Geometry: final body of the model. Coordinates: model frame, mm. Face numbers are marked on the shaded views. Give positions to 0.01 mm unless a question says otherwise; leave off trailing zeros. Loops run counter-clockwise (first coordinate to the right, second up) from the corner with the lowest first, then second, coordinate; pieces in that order, holes last.
from build123d import *

# Parameters (mm, degrees)
SKETCH1_R          = 88.5571
SKETCH1_R_2        = 72.5043
SKETCH3_R          = 84.1375
CUT_EXTRUDE1_DEPTH = 44.45
SKETCH4_R          = 84.1375
CUT_EXTRUDE2_DEPTH = 44.45


with BuildPart() as part:
    # Sweep1: sweep along a path in Sketch2
    with BuildLine(Plane.XY) as sweep1_path:
        Line((0, 0), (50.8, 0))
        ThreePointArc((50.8, 0), (142.847625241, -38.127374759), (180.975, -130.175))
        Line((180.975, -130.175), (180.975, -180.975))
    # Sketch1 → Sweep1 (sweep)
    with BuildSketch(Plane(origin=(0, 0, 0), x_dir=(0, 0, -1), z_dir=(1, 0, 0))):
        Circle(SKETCH1_R)
        Circle(SKETCH1_R_2, mode=Mode.SUBTRACT)
    sweep(path=sweep1_path.line)

    # Sketch3 → Cut-Extrude1 (cut)
    with BuildSketch(Plane(origin=(0, -180.975, 0), x_dir=(-1, 0, 0), z_dir=(0, -1, 0))):
        with Locations((-180.975, 0)):
            Circle(SKETCH3_R)
    extrude(amount=-CUT_EXTRUDE1_DEPTH, mode=Mode.SUBTRACT)

    # Sketch4 → Cut-Extrude2 (cut)
    with BuildSketch(Plane.ZY):
        Circle(SKETCH4_R)
    extrude(amount=-CUT_EXTRUDE2_DEPTH, mode=Mode.SUBTRACT)


solid = part.part
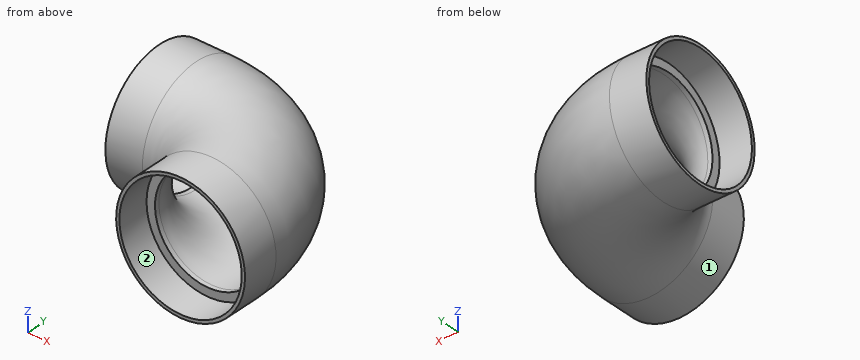
Item 1: Pin query (flat end, axial travel): pin 1 (2 mm diameter, centred on x = 38.5, y = -32.5, fed in from -Z); pin 2 (1.5 mm diameter, centred on x = 199, z = 55, fed in from +Y); pin 3 (4 mm diameter, centred on x = 162, z = 22, fed in from +Y). Return the tip coordinate at first contact, or that it passes through.
Values follow:
pin 1: stops at z = -82.77
pin 2: stops at y = 4.71
pin 3: stops at y = 56.27
Item 2: Draft query along Z for the marked faces 1 and 2. Return one class per face: +Z half, -Z half, draft (parallel to the pull), parting line (faces both ways), or undercut.
Values follow:
face 1: parting line
face 2: undercut
Item 3: Section query B-B on z = -5.5. Return loops of the section in (x, y) (3 decimals), plus the area to 3 significant figures.
Values follow:
outline: (0, -88.386) - (50.8, -88.386) arc R41.789 cw to (92.589, -130.175) - (92.589, -180.975) - (97.017, -180.975) - (97.017, -136.525) - (108.68, -136.525) - (108.68, -130.175) arc R57.88 ccw to (50.8, -72.295) - (44.45, -72.295) - (44.45, -83.958) - (0, -83.958) - close; (0, 83.958) - (44.45, 83.958) - (44.45, 72.295) - (50.8, 72.295) arc R202.47 cw to (253.27, -130.175) - (253.27, -136.525) - (264.933, -136.525) - (264.933, -180.975) - (269.361, -180.975) - (269.361, -130.175) arc R218.561 ccw to (50.8, 88.386) - (0, 88.386) - close
area: 7,780 mm2
Item 4: Ray query, probe 1 along Y at (x, z) = (46.25, 0); probe 2 along Y at (x, z) = (34, 0); probe 3 along X at (y, z) = (-131.75, 0). Return the intervals inside material, ascending.
Values follow:
probe 1: y = -88.56 to -72.5, 72.5 to 88.56
probe 2: y = -88.56 to -84.14, 84.14 to 88.56
probe 3: x = 92.42 to 108.47, 253.48 to 269.53
Item 5: Section query A-A on z = -52.5. Return loops of the section in (x, y) (3 decimals).
Values follow:
outline: (0, -71.317) - (50.8, -71.317) arc R58.858 cw to (109.658, -130.175) - (109.658, -180.975) - (115.226, -180.975) - (115.226, -136.525) - (130.969, -136.525) - (130.969, -130.175) arc R80.169 ccw to (50.8, -50.006) - (44.45, -50.006) - (44.45, -65.749) - (0, -65.749) - close; (0, 65.749) - (44.45, 65.749) - (44.45, 50.006) - (50.8, 50.006) arc R180.181 cw to (230.981, -130.175) - (230.981, -136.525) - (246.724, -136.525) - (246.724, -180.975) - (252.292, -180.975) - (252.292, -130.175) arc R201.492 ccw to (50.8, 71.317) - (0, 71.317) - close
